Autodesk Inventor part; units mm, degrees
ref_plane "XZ Plane" through (0, 0, 0) normal (0, 1, 0) x (-1, 0, 0)
ref_plane "Work Plane1" through (0, 0, 0) normal (0.7071, 0, 0.7071) x (0, -1, 0)
sketch "Sketch1" plane through (0, 0, 0) normal (0.7071, 0, 0.7071) x (0, -1, 0)
  line L0 (-9, 0) -> (-9, 10)
  line L1 (-9, 10) -> (-4, 10)
  line L2 (-4, 10) -> (-4, 0)
  line L3 (-4, 0) -> (0, 0)
  line L4 (0, 0) -> (0, 13)
  line L5 (0, 13) -> (49, 73)
  line L6 (49, 73) -> (49, 82.7959)
  line L7 (49, 82.7959) -> (44, 82.7959)
  line L8 (44, 82.7959) -> (-13, 13)
  line L9 (-13, 13) -> (-13, 0)
  line L10 (-13, 0) -> (-9, 0)
  line L11 (0, -16.5592) -> (0, 99.3551)
  line L12 (0, 0) -> (-5.3698, 0) construction
  dimension "d0" = 4
  dimension "d1" = 4
  dimension "d2" = 5
  dimension "d3" = 10
  dimension "d4" = 3
  dimension "d5" = 60
  dimension "d6" = 5
  dimension "d8" = 53
extrude "Extrusion1" add sketch "Sketch1" along normal blind 10
sketch "Sketch2" plane through (0, 13, 0) normal (0, 1, 0) x (0.7071, 0, 0.7071)
  circle A0 centre (5, 5) radius 2.55
  line L0 (0, 0) -> (0, 10)
  line L1 (0, 5) -> (5, 0)
  line L2 (0, 0) -> (10, 0)
  line L3 (5, 0) -> (10, 5)
  line L4 (10, 13) -> (10, 0)
  line L5 (2.5, 2.5) -> (5, 5) construction
  line L6 (5, 5) -> (7.5, 2.5) construction
  dimension "d11" = 5.1
  dimension "d12" = 45
  dimension "d13" = 45
extrude "Extrusion2" cut sketch "Sketch2" against normal through all
fillet "Fillet1" radius 2 2 edges at (3.5355, 2, 3.5355) (3.5355, 11, 3.5355)
properties part number "Foot thing"
Input: part model. Units: mm. Frame: model coordinates. A direction names the side the tool comes from. Give positions to 0.01 mm unless a question says otherwise; leave off trailing zeros. Write each loop counter-clockwise with the first axis right and the second up, starting at its lowest first coordinate (ties: lowest second). Pieces come first, ordered by that corner, then holes. Notation, with made-up numbers: M 78,23 L 91,23 A17 cw 91,38 Z; hole C 61.5,70.5 d2. An arc over 180 degrees is marked long. Write item = value, one per line. Start each with the question number.
1) Draft query along Y for faces 4 (the flat face through (8, 9, -3)), 5 (the cylindrical face through (4.14, 1.97, 2.97)), 6 (the flat face through (33.595, -24.157, -26.623)). Return one class per face: +Y half, -Y half, draft (parallel to the pull), parting line (faces both ways), or undercut.
2) First-contact query: pin 1 Ø6 at (x, z) = (7.07, 0) entering from -Y; pin 2 Ø10 at (y, z) = (-3.5, -35) entering from +X; pin 3 Ø1 at (x, z) = (20.5, -9) entering from -Y. Flat tips, straight axial feed; report the tip coordinate or a pass-through.
3) Cut plane B-B on z = -33. Return the cut outline in (x, y), then the cut area to 3 significant figures.
4) Cut plane A-A on x = 33. Return the cut outline in (y, z), then the cut area to 3 significant figures.
5) Material intervals for line 1 along X through (y, z) = (1.65, 0); line 2 along X through (y, z) = (-39, -48.5); line 3 along Z through (x, y) = (57, -42), sorted ascending. Write a range as [from, to].
6) Reachability of faces 1 (the flat face through (10.557, 6.535, -3.585)), 2 (the cylindrical face through (4.14, 10.97, 2.97)), 3 (the flat face through (9, 0, -2)) from +Z, -Z, +X, -X, +Y, -Y: full face, straight path, thin tool, end or side. Return the list, or none.
Solved:
q1.face_4 = undercut
q1.face_5 = draft
q1.face_6 = -Y half
q2.pin_1 = 0
q2.pin_2 = through
q2.pin_3 = -6.83
q3.outline = M 33,-27.5 L 47.14,-35.66 L 47.14,-22.66 L 33,-14.5 Z
q3.area = 184 mm2
q4.outline = M -27.5,-33 L -14.5,-33 L -6.33,-18.86 L -19.33,-18.86 Z
q4.area = 184 mm2
q5.line_1 = [3.54, 4.52], [9.62, 14.14]
q5.line_2 = [48.5, 59.93]
q5.line_3 = [-56.63, -42.86]
q6.face_1 = +Z, -X
q6.face_2 = +Z, -X, +Y, -Y
q6.face_3 = +Z, -X, -Y
